Solid Edge part; units mm, degrees
sketch "Sketch1" plane through (0, 0, 0) normal (0, 0, 1) x (1, 0, 0)
  line L0 (0, 58.5) -> (0, 6.5)
  line L1 (13, 6.5) -> (13, 58.5)
  arc A0 (13, 6.5) -> (0, 6.5) centre (6.5, 6.5) cw
  arc A1 (0, 58.5) -> (13, 58.5) centre (6.5, 58.5) cw
extrude "Protrusion1" add sketch "Sketch1" along normal blind 6.5
sketch "Sketch2" plane through (6.5, 0, 0) normal (1, 0, 0) x (0, 1, 0)
  line L0 (3.5, 5.5) -> (3.5, 6.5)
  line L1 (3.5, 6.5) -> (6.5, 6.5)
  line L2 (6.5, 1) -> (6.5, 6.5)
  line L3 (3.5, 1) -> (6.5, 1)
  line L4 (3.5, 1) -> (2.6811, 3.25)
  line L5 (3.5, 5.5) -> (2.6811, 3.25)
revolve "RevolvedCutout1" cut sketch "Sketch2" angle 360 about axis through (6.5, 6.5, 1) along (0, 0, 1)
chamfer "Chaflán_38" distance 0.75 angle 45 1 edges at (6.5, 3.5, 6.5)
pattern_linear "Pattern1" count 5 spacing 13 along (0, 1, 0) of "RevolvedCutout1", "Chaflán_38"
chamfer "Chaflán_39" distance 1.5 angle 45 8 edges at (13, 32.5, 6.5) (6.5, 0, 6.5) (0, 32.5, 6.5) (6.5, 65, 6.5) (13, 32.5, 0) (6.5, 0, 0) (0, 32.5, 0) (6.5, 65, 0)
Could you check a few things on this model? Use its own coordinates, in mm. A direction names the side the tool comes from. Coordinates: 2 decimals unless noted, no trailing zeros. Order: outer loops, then holes, each group sorted by start corner. A loop starts at its lowest first (then second) coordinate and runs counter-clockwise, first axis right, second up.
Q1. Thinking about a two-plate mould opening in Y: for faces 4 (the flat face through (12, 32, 6)), 5 (the conical face through (8.357, 8.921, 5.359)), 6 (the conical face through (6.4, 63.8, 6.2)), which applies, released by +Y, released by -Y, zero draft, split by the parting line, or undercut?
Q2. Suppose I cut it at A-A on y = 27.5. Please give me the cut outline in (x, z), and give its area (3 significant figures).
Q3. Please list where these lines run through material, in increasing order: L1, parallel to Y at x = 7, z = 1.5; L2, parallel to Y at x = 6, z = 3.5; L3, parallel to X at y = 31.5, z = 6.
Q4. Suppose I cut it at B-B on y = 19.5. Please give me the cut outline in (x, z).
Q5. Which directions (+Z, -Z, +X, -X, +Y, -Y) give clear straight access to the entire face, cutting with the end or side of a thin tool? Please do faces 1 (the conical face through (6.4, 1.2, 0.3)), 2 (the flat face through (7, 33, 1)), 3 (the conical face through (7.669, 42.681, 5.359)).
Q6. Will this pin go through, and if not, where does the flat tip stop? pin 1 (3.5 mm diameter, centred on x = 6.5, y = 6.5, fed in from +Z).
Answer:
1. face 4: zero draft
1. face 5: undercut
1. face 6: released by +Y
2. outline: (0, 1.5) - (1.5, 0) - (11.5, 0) - (13, 1.5) - (13, 5) - (11.5, 6.5) - (1.5, 6.5) - (0, 5) - close
2. area: 80.0 mm2
3. L1: y = 0.02 to 3.36, 9.64 to 16.36, 22.64 to 29.36, 35.64 to 42.36, 48.64 to 55.36, 61.64 to 64.98
3. L2: y = 0.02 to 2.81, 10.19 to 15.81, 23.19 to 28.81, 36.19 to 41.81, 49.19 to 54.81, 62.19 to 64.98
3. L3: x = 1 to 3.41, 9.59 to 12
4. outline: (0, 1.5) - (1.5, 0) - (11.5, 0) - (13, 1.5) - (13, 5) - (11.5, 6.5) - (10.25, 6.5) - (9.5, 5.75) - (9.5, 5.5) - (10.32, 3.25) - (9.5, 1) - (3.5, 1) - (2.68, 3.25) - (3.5, 5.5) - (3.5, 5.75) - (2.75, 6.5) - (1.5, 6.5) - (0, 5) - close
5. face 1: -Z, -Y
5. face 2: +Z
5. face 3: none
6. pin 1: stops at z = 1
